Source: CAD feature listing. Evaluate the final solid. Frame: model axes, mm. Face numbers are marked on the shaded views. A direction names the side the tool comes from. Round coordinates to 2 decimals unless told otherwise and drop trailing zeros. Order: outer loops, then holes, each group sorted by start corner. A loop starts at its lowest first (then second) coordinate and runs counter-clockwise, first axis right, second up. Notation, with made-up numbers: (-17.75, 53.5) -> (10.25, 53.5) arc R19 ccw to (10.25, 68.5) -> close; hole circle Ø2 at (-25, 84). An arc over 180 degrees is marked (long way). One line per item, written item: value. Start each with the question number.
1) Mould query, pull axis Y, two halves, no side actions, for the marked faces 1, 2 and 3. Classes: pulls with the +Y half, pulls with the -Y half, needs draft (parallel to the pull), parting line crosses it, or undercut.
2) Pin query (flat end, axial travel): P1, Ø3, axis at x = 43, y = 85.5, coming from the +Z side; P2, Ø5, axis at x = 21.5, y = -9.5, coming from the -Z side; P3, Ø2, axis at x = -7.5, z = 5, coming from the -Y side. Return the tip coordinate at first contact, or that it passes through.
3) Section C-C (y = 25.5). Return the cut outline in (x, z).
4) Ray query, L1, parallel to Y at x = 49, z = 6.5 (3 decimals); L2, parallel to X at y = 81, z = -9.5; L3, parallel to Z at x = -13, y = 37. Return the intervals inside material, ascending.
5) Section D-D (z = 4). Return the cut outline in (x, y) (3 decimals).
6) Reachability of the marked faces 4 and 5 from +Z, -Z, +X, -X, +Y, -Y: full face, straight path, thin tool, end or side. Return the list, or none.
7) Section B-B (x = 44.5). Return the cut outline in (y, z) (3 decimals), and give its area (3 significant figures).
8) Section A-A (z = -7). Return the cut outline in (x, y) (3 decimals), and give its area (3 significant figures).
```python
from build123d import *

# Parameters (mm, degrees)
F0_W      = 97.79
F0_H      = 45.72
F1_DEPTH  = 101.6
F2_W      = 91.44
F2_H      = 95.25
F3_DEPTH  = 44.45
F4_W      = 19.05
F4_H      = 6.35
F5_ANGLE  = 180
F7_DEPTH  = 25.4
F8_R      = 3.17499
F10_D     = 6.35
F10_DEPTH = 101.601


# Not quite as in the source:
# - a fillet or chamfer is up to 0.001 mm smaller than in the source, because OpenCascade refuses the exact size


with BuildPart() as f1:
    # F0 (on Front) → F1 (new body)
    with BuildSketch(Plane.XZ):
        with Locations((15.4838143581, 4.6649015626)):
            Rectangle(F0_W, F0_H)
    extrude(amount=-F1_DEPTH)

    # F2 (on face) → F3 (cut)
    with BuildSketch(Plane.XY.offset(27.5249015626)):
        with Locations((15.4838143581, 50.8)):
            Rectangle(F2_W, F2_H)
    extrude(amount=-F3_DEPTH, mode=Mode.SUBTRACT)

    # F4 (on face) → F5 (revolve)
    with BuildSketch(Plane.XZ):
        with Locations((5.9588143581, 6.8874015626)):
            Rectangle(F4_W, F4_H)
        with Locations((5.9588143581, 0.5374015626)):
            Rectangle(F4_W, F4_H)
    revolve(axis=Axis((15.4838143581, 0, 3.7124015626), (0, 0, 1)), revolution_arc=F5_ANGLE)

    # F6 (on face) → F7 (cut)
    with BuildSketch(Plane.XY.offset(10.0624015626)):
        with BuildLine():
            Line((28.1838143581, 0), (2.7838143581, 0))
            ThreePointArc((2.7838143581, 0), (15.4838143581, -12.7), (28.1838143581, 0))
        make_face()
    extrude(amount=-F7_DEPTH, mode=Mode.SUBTRACT)

    # F8 (radius 3.175 in the source; OpenCascade refuses exactly that, so slightly less here)
    f8_edges = [f1.edges().sort_by_distance(p)[0] for p in [
        (15.483814, -19.05, 10.062402),
        (15.483814, -12.7, 10.062402),
        (15.483814, -19.05, -2.637598),
        (15.483814, -12.7, -2.637598),
    ]]
    fillet(f8_edges, radius=F8_R)

    # F10 (through all, one way)
    with BuildSketch(Plane.XZ):
        with Locations((14.5096713677, 2.1249015626)):
            Circle(F10_D / 2)
    extrude(amount=-F10_DEPTH, mode=Mode.SUBTRACT)


solid = f1.part
```
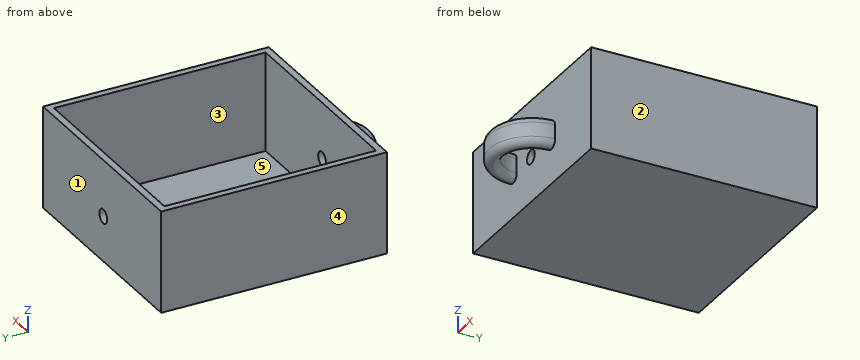
Findings:
1. face 1: pulls with the +Y half
1. face 2: needs draft
1. face 3: undercut
2. P1: z = -16.93
2. P2: z = -1.82
2. P3: y = 0
3. outline: (-33.41, -18.2) -> (64.38, -18.2) -> (64.38, 27.52) -> (61.2, 27.52) -> (61.2, -16.93) -> (-30.24, -16.93) -> (-30.24, 27.52) -> (-33.41, 27.52) -> close
4. L1: 0 to 3.175, 98.425 to 101.6
4. L2: -33.41 to -30.24, 61.2 to 64.38
4. L3: -18.2 to -16.93
5. outline: (-33.411, 0) -> (-3.566, 0) arc R19.05 ccw to (34.534, 0) -> (64.379, 0) -> (64.379, 101.6) -> (17.072, 101.6) -> (17.072, 98.425) -> (61.204, 98.425) -> (61.204, 3.175) -> (17.072, 3.175) -> (17.072, 0) -> (28.184, 0) arc R12.7 cw to (2.784, 0) -> (11.948, 0) -> (11.948, 3.175) -> (-30.236, 3.175) -> (-30.236, 98.425) -> (11.948, 98.425) -> (11.948, 101.6) -> (-33.411, 101.6) -> close
6. face 4: +Z, -Z, -X, +Y, -Y
6. face 5: +Z
7. outline: (0, -18.195) -> (101.6, -18.195) -> (101.6, 27.525) -> (98.425, 27.525) -> (98.425, -16.925) -> (3.175, -16.925) -> (3.175, 27.525) -> (0, 27.525) -> close
7. area: 411 mm2
8. outline: (-33.411, 0) -> (64.379, 0) -> (64.379, 101.6) -> (-33.411, 101.6) -> close; hole (-30.236, 3.175) -> (61.204, 3.175) -> (61.204, 98.425) -> (-30.236, 98.425) -> close
8. area: 1,230 mm2
